Work out the finished part from the listing and answer in its coordinate system (mm). A direction names the side the tool comes from. Coordinates: 2 decimals unless noted, no trailing zeros. Loops run counter-clockwise (first coordinate to the right, second up) from the corner with the lowest first, then second, coordinate; pieces in that order, holes last. Notation, with made-up numbers: (2, 5.5) -> (60, 5.5) arc R20 ccw to (60, 19.5) -> close; hole circle Ø7 at (6.25, -1). An arc over 180 degrees is marked (long way). Use a Markdown table: item, result.
from build123d import *

# Parameters (mm, degrees)
BOSS_EXTRUDE1_DEPTH = 1.499997
SKETCH3_R           = 3.81
SKETCH3_R_2         = 1.5
BOSS_EXTRUDE2_DEPTH = 1.499997
BOSS_EXTRUDE3_DEPTH = 2.999994
FILLET1_R           = 3.175


with BuildPart() as part:
    # Sketch2 → Boss-Extrude1 (new, symmetric)
    with BuildSketch(Plane(origin=(0, 0, 0), x_dir=(0, 0, -1), z_dir=(1, 0, 0))):
        Polygon((-19.672783942, -4.025738686), (13.322783942, 15.024261314), (19.672783942, 4.025738686), (-13.322783942, -15.024261314), align=None)
        Polygon((-16.021265259, -5.730354569), (-12.973265259, -11.009645431), (-10.375189048, -9.509645431), (-13.423189048, -4.230354569), align=None, mode=Mode.SUBTRACT)
        Polygon((10.375189048, 9.509645431), (13.423189048, 4.230354569), (16.021265259, 5.730354569), (12.973265259, 11.009645431), align=None, mode=Mode.SUBTRACT)
    extrude(amount=BOSS_EXTRUDE1_DEPTH, both=True)



with BuildPart() as body_2:
    # Sketch3 → Boss-Extrude2 (new, symmetric)
    with BuildSketch(Plane(origin=(0, 0, 0), x_dir=(0, 0, -1), z_dir=(1, 0, 0))):
        with Locations((-25.4, 7.62)):
            Circle(SKETCH3_R)
        with Locations((-25.4, 7.62)):
            Circle(SKETCH3_R_2, mode=Mode.SUBTRACT)
    extrude(amount=BOSS_EXTRUDE2_DEPTH, both=True)


with BuildPart() as part_1:
    add(part.part)

    add(body_2.part)  # Boss-Extrude3 merges body 2
    # Sketch4 → Boss-Extrude3 (add)
    with BuildSketch(Plane(origin=(1.499997, 0, 0), x_dir=(0, 0, -1), z_dir=(1, 0, 0))):
        with BuildLine():
            Line((-28.458311324, 5.347813422), (-13.322783942, -15.024261314))
            Line((-13.322783942, -15.024261314), (-19.672783942, -4.025738686))
            Line((-19.672783942, -4.025738686), (-8.640886423, 2.343530316))
            Line((-8.640886423, 2.343530316), (-23.495, 10.919556788))
            ThreePointArc((-23.495, 10.919556788), (-22.100443212, 9.525), (-21.59, 7.62))
            ThreePointArc((-21.59, 7.62), (-24.203351794, 4.002800383), (-28.458311324, 5.347813422))
        make_face()
    extrude(amount=-BOSS_EXTRUDE3_DEPTH)

    # Fillet1
    fillet1_edges = [part_1.edges().sort_by_distance(p)[0] for p in [
        (0, 2.343530316, 8.640886423),
        (0, 15.024261314, -13.322783942),
        (0, 4.025738686, -19.672783942),
        (0, -15.024261314, 13.322783942),
    ]]
    fillet(fillet1_edges, radius=FILLET1_R)


solid = part_1.part
Q1. Determine the mould class of faces 3 (the cylindrical face through (-0.021, 13.745, -13.016)), 4 (the flat face through (0.021, 7.036, 16.769)), 5 (the flat face through (1.5, 0, 6)), 6 (the cylindrical face through (-0.021, 4.332, -18.393)) for opening direction Z: pulls with the +Z half, pulls with the -Z half, needs draft (parallel to the pull), parting line crosses it, or undercut.
Solved:
| item | result |
|---|---|
| face 3 | parting line crosses it |
| face 4 | undercut |
| face 5 | needs draft |
| face 6 | pulls with the -Z half |
Q2. Section C-C on z = 25.4 is taken. Determine the outline of the cut face in (x, y).
Solved:
| item | result |
|---|---|
| outline | (-1.5, 1.23) -> (1.5, 1.23) -> (1.5, 6.12) -> (-1.5, 6.12) -> close; (-1.5, 9.12) -> (1.5, 9.12) -> (1.5, 11.43) -> (-1.5, 11.43) -> close |
Q3. Consider line 1 (Z direction, x = -1.2, y = 6.75); line 2 (Y direction, x = -0.1, z = 25.4); line 3 (Y direction, x = 1.3, z = 9.5). Determine where each line is inside the solid, lowest interval first. Write a range as [from, to].
Solved:
| item | result |
|---|---|
| line 1 | [-18.1, -15.43], [-11.97, 1.01], [16.27, 24.18], [26.62, 29.11] |
| line 2 | [1.23, 6.12], [9.12, 11.43] |
| line 3 | [-12.82, 2.95] |
Q4. For faces 1 (the cylindrical face through (0.02, -13.96, 13.14)), 2 (the flat face through (0.021, -4.97, 14.704)), determine the directions among +Z, -Z, +X, -X, +Y, -Y from which every point of the face is accessible in a straight line to the end or side of a thin tool.
Solved:
| item | result |
|---|---|
| face 1 | +X, -X, -Y |
| face 2 | +X, -X |
Q5. Section D-D on z = 18 is taken. Determine the outline of the cut face in (x, y), and give its area (3 significant figures).
Solved:
| item | result |
|---|---|
| outline | (-1.5, -8.73) -> (1.5, -8.73) -> (1.5, 7.75) -> (-1.5, 7.75) -> close |
| area | 49.4 mm² |
Q6. Given pin 1 Ø4 at (y, z) = (7.62, 25.4) entering from +X, flat-ended and moving along its own axis, determine where the tip first touches the part or whether it passes through.
Solved:
| item | result |
|---|---|
| pin 1 | x = 1.5 |
Q7. Section A-A on x = 0.9 is taken. State how many separate pieces and enclosed holes the cut face has, and give its area (3 significant figures).
Solved:
| item | result |
|---|---|
| separate pieces | 1 |
| enclosed holes | 3 |
| area | 613 mm² |
Q8. Section B-B on y = 7.62 is taken. Determine the outline of the cut face in (x, z), and give its area (3 significant figures).
Solved:
| item | result |
|---|---|
| outline | (-1.5, -17.6) -> (1.5, -17.6) -> (1.5, -14.93) -> (-1.5, -14.93) -> close; (-1.5, -11.47) -> (1.5, -11.47) -> (1.5, -0.5) -> (-1.5, -0.5) -> close; (-1.5, 17.78) -> (1.5, 17.78) -> (1.5, 23.9) -> (-1.5, 23.9) -> close; (-1.5, 26.9) -> (1.5, 26.9) -> (1.5, 29.21) -> (-1.5, 29.21) -> close |
| area | 66.2 mm² |
